from build123d import *

# Parameters (mm, degrees)
SKETCH1_W           = 19
SKETCH1_H           = 20
BOSS_EXTRUDE1_DEPTH = 8
SKETCH2_W           = 19
SKETCH2_H           = 8
BOSS_EXTRUDE2_DEPTH = 20
SKETCH3_R           = 2
CUT_EXTRUDE1_DEPTH  = 20
SKETCH4_R           = 2
CUT_EXTRUDE2_DEPTH  = 20
BOSS_EXTRUDE3_DEPTH = 19
SKETCH7_R           = 3.5
CUT_EXTRUDE3_DEPTH  = 20
SKETCH8_R           = 3.5
CUT_EXTRUDE4_DEPTH  = 20


with BuildPart() as part:
    # Sketch1 → Boss-Extrude1 (new body)
    with BuildSketch(Plane.XY):
        with Locations((-3.134342089, 6.179897069)):
            Rectangle(SKETCH1_W, SKETCH1_H)
    extrude(amount=BOSS_EXTRUDE1_DEPTH)

    # Sketch2 → Boss-Extrude2 (add)
    with BuildSketch(Plane.XY.offset(8)):
        with Locations((-3.134342089, 12.179897069)):
            Rectangle(SKETCH2_W, SKETCH2_H)
    extrude(amount=BOSS_EXTRUDE2_DEPTH)

    # Sketch3 → Cut-Extrude1 (cut)
    with BuildSketch(Plane.XY.offset(8)):
        with Locations((-8.634342089, 1.179897069)):
            Circle(SKETCH3_R)
        with Locations((2.365657911, 1.179897069)):
            Circle(SKETCH3_R)
    extrude(amount=-CUT_EXTRUDE1_DEPTH, mode=Mode.SUBTRACT)

    # Sketch4 → Cut-Extrude2 (cut)
    with BuildSketch(Plane.XZ.offset(-8.179897069)):
        with Locations(Location((-7.634342089, 21, 0), (0, 0, 270))):
            Circle(SKETCH4_R)
        with Locations(Location((1.365657911, 21, 0), (0, 0, 270))):
            Circle(SKETCH4_R)
    extrude(amount=-CUT_EXTRUDE2_DEPTH, mode=Mode.SUBTRACT)

    # Sketch5 → Boss-Extrude3 (add)
    with BuildSketch(Plane.ZY.offset(12.634342089)):
        Polygon((28, 8.179897069), (8, -3.820102931), (8, 8.179897069), align=None)
    extrude(amount=-BOSS_EXTRUDE3_DEPTH)

    # Sketch7 → Cut-Extrude3 (cut)
    with BuildSketch(Plane(origin=(0, 8.179897069, 0), x_dir=(1, 0, 0), z_dir=(0, 1, 0))):
        with Locations(Location((1.365657911, -21, 0), (0, 0, 180))):
            Circle(SKETCH7_R)
        with Locations(Location((-7.634342089, -21, 0), (0, 0, 180))):
            Circle(SKETCH7_R)
    extrude(amount=-CUT_EXTRUDE3_DEPTH, mode=Mode.SUBTRACT)

    # Sketch8 → Cut-Extrude4 (cut)
    with BuildSketch(Plane(origin=(0, 0, 8), x_dir=(-1, 0, 0), z_dir=(0, 0, -1))):
        with Locations((8.634342089, 1.179897069)):
            Circle(SKETCH8_R)
        with Locations((-2.365657911, 1.179897069)):
            Circle(SKETCH8_R)
    extrude(amount=-CUT_EXTRUDE4_DEPTH, mode=Mode.SUBTRACT)


solid = part.part
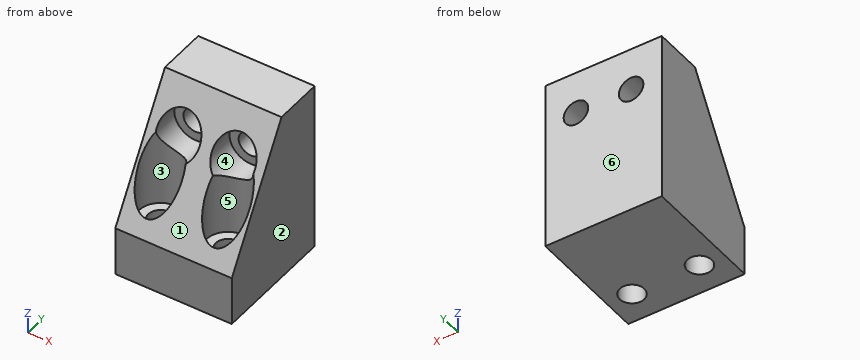
Input: part model. Units: mm. Frame: model coordinates. Face numbers are marked on the shaded views. A direction names the side the tool comes from. Give positions to 0.01 mm unless a question says otherwise; leave off trailing zeros. Write each loop counter-clockwise with the first axis right and the second up, starting at its lowest first coordinate (ties: lowest second). Pieces come first, ordered by that corner, then holes.
Q1. Section D-D, the plane y = 7.75. Output: boundary loops of the cut face in (x, z).
Q2. Section C-C, the plane z = 15.25. Output: boundary loops of the cut face in (x, y).
Q3. Section A-A, the plane z = 21. Output: boundary loops of the cut face in (x, y).
Q4. Material intervals for probe 1 along X at (y, z) = (4.9, 21); probe 2 along X at (y, z) = (2.25, 13.25); probe 3 along Z at (x, y) = (-9.75, -1.5), sorted ascending.
Q5. Section B-B, the plane x = 2.25. Output: boundary loops of the cut face in (y, z).
Q6. Set-up query: the marked faces 4, 5 and 6. Return all of +Z, -Z, +X, -X, +Y, -Y with unobstructed straight access to the full face (end or side cutting, diameter ignored); none if empty.
Q7. Pull-direction query (X, two-part tool) for the marked faces 1, 2 and 3; classes: pulls with the +X half, pulls with the -X half, needs draft (parallel to the pull), parting line crosses it, or undercut.
Q8. First-contact query: P1, Ø3.5, axis at x = 1.37, z = 21, coming from the -Y side; P2, Ø4, axis at x = 2, z = 16.5, coming from the -Y side; P3, Ø3.5, axis at x = -6.5, z = 21.5, coming from the -Y side; P4, Ø1, axis at x = -6.5, y = -0.5, coming from the +Z side. Flat tips, straight axial feed; report the tip coordinate or a pass-through.
Filled in:
1. outline: (-12.63, 0) - (6.37, 0) - (6.37, 27.28) - (-12.63, 27.28) - close; hole circle Ø7 at (-7.63, 21); hole circle Ø7 at (1.37, 21)
2. outline: (-12.63, 0.53) - (-12.07, 0.53) arc R3.5 cw (long way) to (-5.2, 0.53) - (-1.07, 0.53) arc R3.5 cw (long way) to (5.8, 0.53) - (6.37, 0.53) - (6.37, 16.18) - (-12.63, 16.18) - close
3. outline: (-12.63, 3.98) - (-11.13, 3.98) - (-11.13, 8.18) - (-9.63, 8.18) - (-9.63, 16.18) - (-12.63, 16.18) - close; (-5.63, 8.18) - (-4.13, 8.18) - (-4.13, 3.98) - (-2.13, 3.98) - (-2.13, 8.18) - (-0.63, 8.18) - (-0.63, 16.18) - (-5.63, 16.18) - close; (3.37, 8.18) - (4.87, 8.18) - (4.87, 3.98) - (6.37, 3.98) - (6.37, 16.18) - (3.37, 16.18) - close
4. probe 1: x = -12.63 to -11.13, -4.13 to -2.13, 4.87 to 6.37
4. probe 2: x = -12.63 to -11.97, -5.3 to -0.97, 5.7 to 6.37
4. probe 3: z = 0 to 8
5. outline: (-3.82, 0) - (-0.82, 0) - (-0.82, 8) - (-2.32, 8) - (-2.32, 10.5) - (-3.82, 8) - close; (3.18, 0) - (16.18, 0) - (16.18, 19.21) - (8.18, 19.21) - (8.18, 17.61) - (4.68, 17.61) - (4.68, 8) - (3.18, 8) - close; (6.01, 24.39) - (8.18, 24.39) - (8.18, 22.79) - (16.18, 22.79) - (16.18, 28) - (8.18, 28) - close
6. face 4: -Y
6. face 5: +Z
6. face 6: +Z, -Z, +X, -X, +Y
7. face 1: needs draft
7. face 2: pulls with the +X half
7. face 3: undercut
8. P1: passes through
8. P2: stops at y = 3.76
8. P3: stops at y = 8.18
8. P4: stops at z = 8
